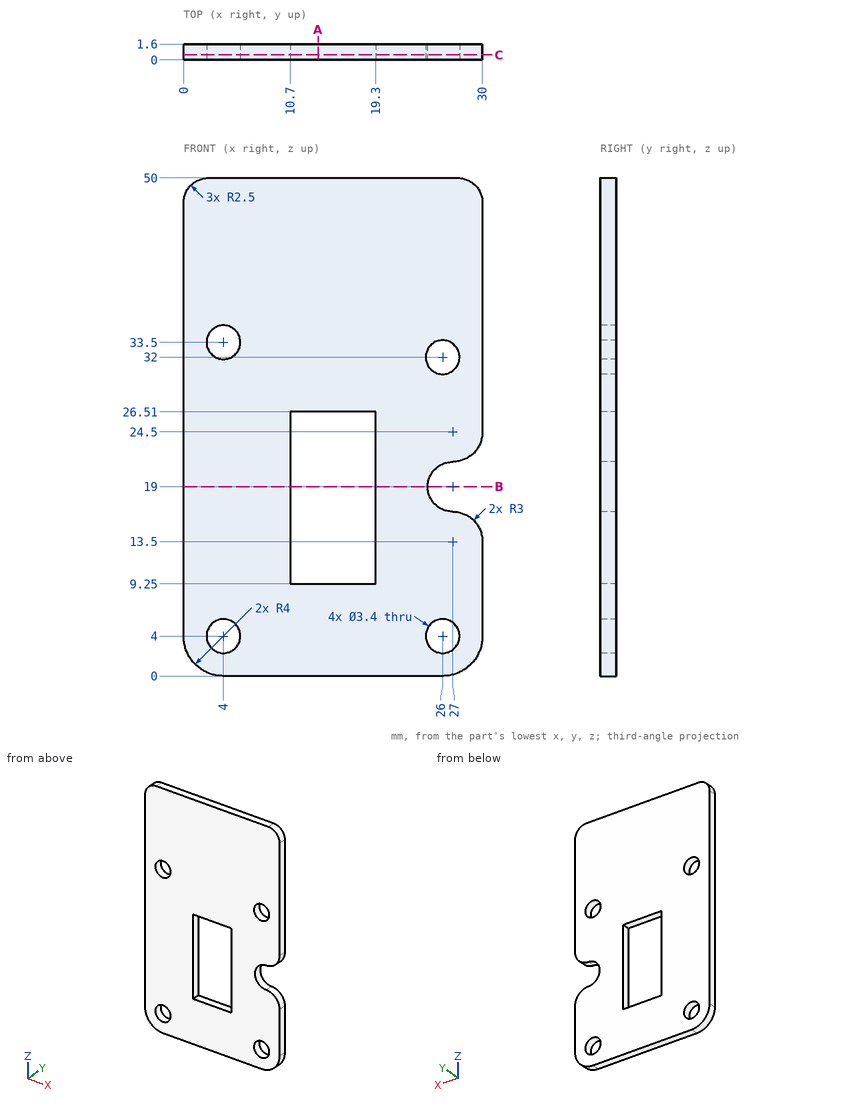
For this review, use the dimensioned drawing (mm, ordinates from the lowest corner) and the shaded views. Coordinates: 2 decimals unless noted, no trailing zeros. Write each loop counter-clockwise with the first axis right and the second up, starting at its lowest first coordinate (ties: lowest second). Pieces come first, ordered by that corner, then holes. Notation, with made-up numbers: (65, 72.5) - (110, 72.5) arc R33 ccw to (110, 103.5) - close; hole circle Ø6 at (54, 72.5). An arc over 180 degrees is marked (long way). Answer as a JSON object with one key per item and string values. Group by question number.
1. Add section C-C (y = 0.5). Give the boundary of the cut face in (x, z), plus the area to 3 significant figures.
2. Add section A-A (x = 13.5). Give the boundary of the cut face in (y, z).
3. Add section B-B (z = 19). Give the boundary of the cut face in (x, y).
4. Clearance check with a flat-ended pin moving along its axis: pin 1 Ø2.5 at (x, z) = (26, 4) entering from +Y. State where the tip first meets the part, or that it passes through.
5. To check wall thickness, follow probe 1 along X at (y, z) = (0.75, 4); probe 2 along Z at (x, y) = (4, 1); probe 3 along Z at (x, y) = (26, 0.7). State the ranges of each line that lie inside material, in increasing order.
Findings:
{
 "1": {"outline": "(0, 4) arc R4 ccw to (4, 0) - (26, 0) arc R4 ccw to (30, 4) - (30, 13.5) arc R3 ccw to (27, 16.5) arc R2.5 cw to (27, 21.5) arc R3 ccw to (30, 24.5) - (30, 47.5) arc R2.5 ccw to (27.5, 50) - (2.5, 50) arc R2.5 ccw to (0, 47.5) - close; hole circle Ø3.4 at (4, 4); hole circle Ø3.4 at (4, 33.5); hole (10.7, 9.25) - (19.3, 9.25) - (19.3, 26.51) - (10.7, 26.51) - close; hole circle Ø3.4 at (26, 4); hole circle Ø3.4 at (26, 32)", "area": "1,280 mm²"},
 "2": {"outline": "(0, 0) - (1.6, 0) - (1.6, 9.25) - (0, 9.25) - close; (0, 26.51) - (1.6, 26.51) - (1.6, 50) - (0, 50) - close"},
 "3": {"outline": "(0, 0) - (10.7, 0) - (10.7, 1.6) - (0, 1.6) - close; (19.3, 0) - (24.5, 0) - (24.5, 1.6) - (19.3, 1.6) - close"},
 "4": {"pin 1": "through"},
 "5": {"probe 1": "0 to 2.3, 5.7 to 24.3, 27.7 to 30", "probe 2": "0 to 2.3, 5.7 to 31.8, 35.2 to 50", "probe 3": "0 to 2.3, 5.7 to 16.71, 21.29 to 30.3, 33.7 to 50"}
}
